Can you work these out from the drawing? Everything is in mm from the part's minimum corner. Give positions to 0.01 mm unless a question says otherwise; leave off trailing zeros. Order: outer loops, then holes, each group sorted by start corner. A loop starts at its lowest first (then second) coordinate and runs counter-clockwise, first axis right, second up. Notation, with made-up numbers: M 56.25,-40 L 92.25,-40 A37 cw 92.25,-2 Z; hole C 83.25,14.25 d3. An arc over 180 degrees is marked long. Use a Markdown table: item, result. Add a question column.
Item 1: Suppose I cut it at A-A on y = 61.5. Write out the boundary of the cut face in (x, z).
Item 2: Suppose I cut it at D-D on y = 37. Write out the boundary of the cut face in (x, z), plus the area to 4 significant figures.
Item 3: I'm going to push a flat-ended pin straight in: pin 1 Ø6 at (x, y) = (55, 87) entering from -Z. Where does the tip first touch, or does it pass through?
Item 4: Suppose I cut it at C-C on x = 118.5. Write out the boundary of the cut face in (y, z), plus the area to 3 significant figures.
Item 5: If I drill on L1, parallel to Y at x = 61.5, z = 1.2; L2, parallel to Y at x = 60.5, z = 1.8, over which ranges is the centre line in solid material (lowest first)? Write a range as from..to.
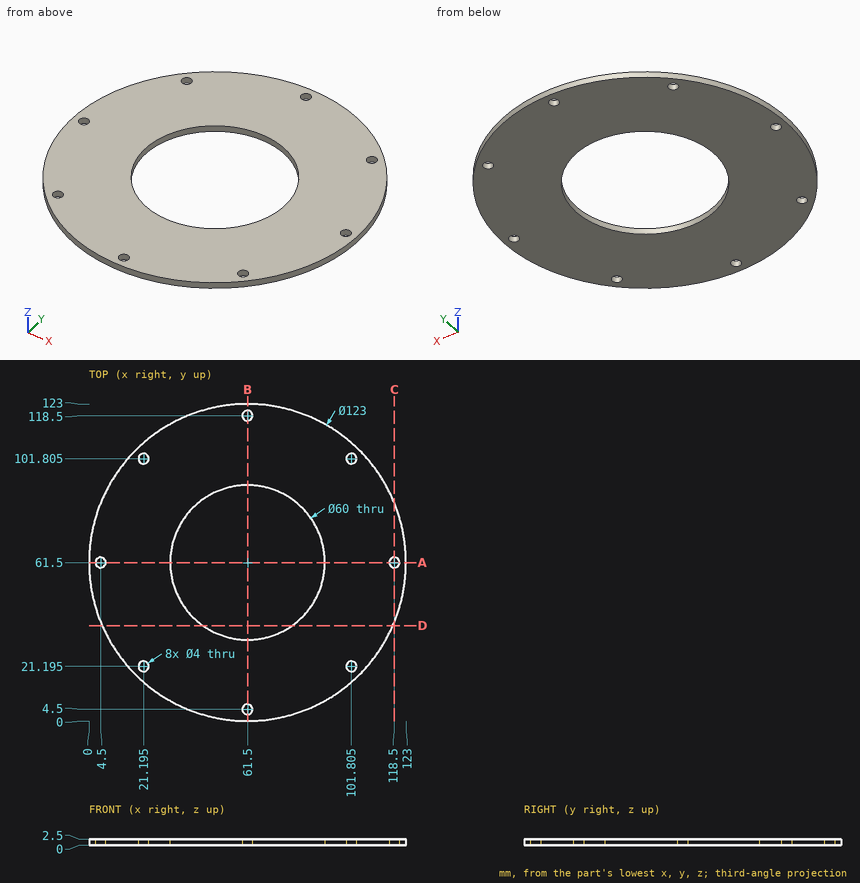
Findings below:
| question | item | result |
|---|---|---|
| 1 | outline | M 0,0 L 2.5,0 L 2.5,2.5 L 0,2.5 Z; M 6.5,0 L 31.5,0 L 31.5,2.5 L 6.5,2.5 Z; M 91.5,0 L 116.5,0 L 116.5,2.5 L 91.5,2.5 Z; M 120.5,0 L 123,0 L 123,2.5 L 120.5,2.5 Z |
| 2 | outline | M 5.09,0 L 44.19,0 L 44.19,2.5 L 5.09,2.5 Z; M 78.81,0 L 117.91,0 L 117.91,2.5 L 78.81,2.5 Z |
| 2 | area | 195.5 mm^2 |
| 3 | pin 1 | passes through |
| 4 | outline | M 38.41,0 L 59.5,0 L 59.5,2.5 L 38.41,2.5 Z; M 63.5,0 L 84.59,0 L 84.59,2.5 L 63.5,2.5 Z |
| 4 | area | 105 mm^2 |
| 5 | L1 | y = 0..2.5, 6.5..31.5, 91.5..116.5, 120.5..123 |
| 5 | L2 | y = 0.01..2.77, 6.23..31.52, 91.48..116.77, 120.23..122.99 |
